from build123d import *

# Parameters (mm, degrees)
F_19_64_0_29688_DIAMETER_HOLE1_D     = 7.540752
F_19_64_0_29688_DIAMETER_HOLE1_DEPTH = 8.382
F_19_64_0_29688_DIAMETER_HOLE1_TIP   = 2.265470457
CHAMFER1_SIZE                        = 0.79375


with BuildPart() as part:
    # Sketch1 → Revolve1 (revolve)
    with BuildSketch(Plane(origin=(0, 0, 0), x_dir=(0, 0, -1), z_dir=(1, 0, 0))):
        Polygon((0, -4.143375), (-6.35, -4.143375), (-6.35, -2.555875), (-5.3721, -2.555875), (-5.3721, 2.613025), (-4.8514, 2.613025), (-4.8514, 3.349625), (-5.3721, 3.349625), (-5.3721, 4.143375), (0, 4.143375), align=None)
    revolve(axis=Axis((0, 0, 0), (0, 1, 0)))

    # 19/64 (0.29688) Diameter Hole1
    with Locations(Plane(origin=(0, 4.143375, 0), x_dir=(1, 0, 0), z_dir=(0, 1, 0))):
        with Locations((0, 0)):
            Hole(F_19_64_0_29688_DIAMETER_HOLE1_D / 2, depth=F_19_64_0_29688_DIAMETER_HOLE1_DEPTH)
            with Locations((0, 0, -(F_19_64_0_29688_DIAMETER_HOLE1_DEPTH + F_19_64_0_29688_DIAMETER_HOLE1_TIP / 2))):  # 118° drill point
                Cone(0, F_19_64_0_29688_DIAMETER_HOLE1_D / 2, F_19_64_0_29688_DIAMETER_HOLE1_TIP, mode=Mode.SUBTRACT)

    # Chamfer1
    chamfer1_edges = [part.edges().sort_by_distance(p)[0] for p in [
        (3.770376, -4.143375, 0),
    ]]
    chamfer(chamfer1_edges, length=CHAMFER1_SIZE)


solid = part.part
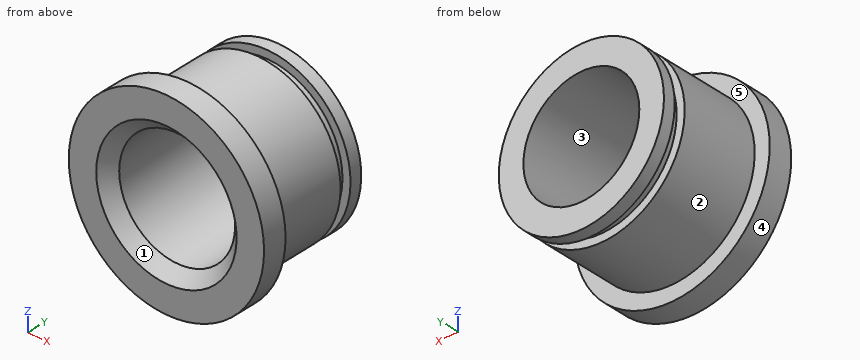
Model file for the job. Use its own axes, mm. Face numbers are marked on the shaded views. A direction names the side the tool comes from. Coordinates: 2 decimals unless noted, no trailing zeros. Write each loop counter-clockwise with the first axis right and the second up, starting at its lowest first coordinate (ties: lowest second). Pieces come first, ordered by that corner, then holes. Notation, with made-up numbers: (44, 40.25) - (72, 40.25) arc R5 cw to (72, 47.25) - close; hole circle Ø1 at (14, 4). An arc over 180 degrees is marked (long way). Write each question's results on one line, items separated by ' | '. Start each with the question number.
1) Cut at A-A (z = 0). Write the cut outline in (x, y).
2) Flat gauge pins, fed straight in: P1, Ø1.5, axis at y = 2.5, z = 3.5, coming from the +X side; P2, Ø3, axis at x = 1, z = -2, coming from the -Y side; P3, Ø2, axis at y = -1, z = 1.5, coming from the +X side. Where does each tip first touch, or does it go through?
3) Mould opens along X. For the marked faces 3, 4 and 5 say: pulls with the +X half, pulls with the -X half, needs draft (parallel to the pull), parting line crosses it, or undercut.
4) 3-axis set-ups, long thin cutter, end or side, ignore diameter. For the marked faces 1 and 2: which of +Z, -Z, +X, -X, +Y, -Y reach the whole face in a straight line?
5) Cut at C-C (y = 0.75). Write the cut outline in (x, z).
6) Cut at B-B (x = 0). Write the cut outline in (y, z).
7) Probe line 1 along X through (y, z) = (-1.25, 0); line 2 along Y through (x, z) = (3.75, -3.25); line 3 along Z through (x, y) = (-1.5, -3). List the from-to ranges inside material, lowest first. Write a range as from..to.
Returned:
1) outline: (-6.35, -4.14) - (-4.56, -4.14) - (-3.77, -3.35) - (-3.77, 4.14) - (-5.37, 4.14) - (-5.37, 3.35) - (-4.85, 3.35) - (-4.85, 2.61) - (-5.37, 2.61) - (-5.37, -2.56) - (-6.35, -2.56) - close; (3.77, -3.35) - (4.56, -4.14) - (6.35, -4.14) - (6.35, -2.56) - (5.37, -2.56) - (5.37, 2.61) - (4.85, 2.61) - (4.85, 3.35) - (5.37, 3.35) - (5.37, 4.14) - (3.77, 4.14) - close
2) P1: x = 4.61 | P2: through | P3: x = 5.35
3) face 3: undercut | face 4: parting line crosses it | face 5: needs draft
4) face 1: -Y | face 2: +Y
5) outline: circle Ø10.74 at (0, 0); hole circle Ø7.54 at (0, 0)
6) outline: (-4.14, -6.35) - (-2.56, -6.35) - (-2.56, -5.37) - (2.61, -5.37) - (2.61, -4.85) - (3.35, -4.85) - (3.35, -5.37) - (4.14, -5.37) - (4.14, -3.77) - (-3.35, -3.77) - (-4.14, -4.56) - close; (-4.14, 4.56) - (-3.35, 3.77) - (4.14, 3.77) - (4.14, 5.37) - (3.35, 5.37) - (3.35, 4.85) - (2.61, 4.85) - (2.61, 5.37) - (-2.56, 5.37) - (-2.56, 6.35) - (-4.14, 6.35) - close
7) line 1: -5.37..-3.77, 3.77..5.37 | line 2: -4.14..2.61, 3.35..4.14 | line 3: -6.17..-3.46, 3.46..6.17
